from build123d import *

# Parameters (mm, degrees)
F0_R     = 7.5
F0_R_2   = 30
F1_DEPTH = 12
F2_R     = 3
F3_DEPTH = 20
F5_DEPTH = 20


with BuildPart() as f1:
    # F0 (on Right) → F1 (new body)
    with BuildSketch(Plane.YZ):
        with BuildLine():
            ThreePointArc((0, 32), (9.372583, 9.372583), (32, 0))
            Line((32, 0), (65, 0))
            ThreePointArc((65, 0), (68.535534, -1.464466), (70, -5))
            Line((70, -5), (70, -8.5))
            Line((70, -8.5), (202, -8.5))
            Line((202, -8.5), (202, 78.5))
            Line((202, 78.5), (70, 78.5))
            Line((70, 78.5), (70, 75))
            ThreePointArc((70, 75), (68.535534, 71.464466), (65, 70))
            Line((65, 70), (32, 70))
            ThreePointArc((32, 70), (9.372583, 60.627417), (0, 38))
            Line((0, 38), (0, 32))
        make_face()
        with Locations((32.5, 35)):
            Circle(F0_R, mode=Mode.SUBTRACT)
        with Locations((142, 35)):
            Circle(F0_R_2, mode=Mode.SUBTRACT)
    extrude(amount=F1_DEPTH)

    # F2 (on face) → F3 (cut)
    with BuildSketch(Plane.XY.offset(78.5)):
        with Locations((6, 80)):
            Circle(F2_R)
        with Locations((6, 110)):
            Circle(F2_R)
        with Locations((6, 140)):
            Circle(F2_R)
        with Locations((6, 170)):
            Circle(F2_R)
    extrude(amount=-F3_DEPTH, mode=Mode.SUBTRACT)

    # F4 (on face) → F5 (cut)
    with BuildSketch(Plane(origin=(0, 0, -8.5), x_dir=(1, 0, 0), z_dir=(0, 0, -1))):
        with BuildLine():
            ThreePointArc((6, -167), (3, -170), (6, -173))
            Line((6, -173), (6, -167))
        make_face()
        with BuildLine():
            ThreePointArc((6, -77), (3, -80), (6, -83))
            Line((6, -83), (6, -80))
            Line((6, -80), (6, -77))
        make_face()
        with BuildLine():
            Line((6, -80), (6, -83))
            ThreePointArc((6, -83), (8.12132, -82.12132), (9, -80))
            Line((9, -80), (6, -80))
        make_face()
        with BuildLine():
            ThreePointArc((6, -107), (3, -110), (6, -113))
            Line((6, -113), (6, -110))
            Line((6, -110), (6, -107))
        make_face()
        with BuildLine():
            Line((6, -110), (6, -113))
            ThreePointArc((6, -113), (8.12132, -112.12132), (9, -110))
            ThreePointArc((9, -110), (8.12132, -107.87868), (6, -107))
            Line((6, -107), (6, -110))
        make_face()
        with BuildLine():
            ThreePointArc((6, -137), (3, -140), (6, -143))
            Line((6, -143), (6, -137))
        make_face()
        with BuildLine():
            Line((6, -137), (6, -143))
            ThreePointArc((6, -143), (8.12132, -142.12132), (9, -140))
            ThreePointArc((9, -140), (8.12132, -137.87868), (6, -137))
        make_face()
        with BuildLine():
            Line((6, -167), (6, -173))
            ThreePointArc((6, -173), (8.12132, -172.12132), (9, -170))
            ThreePointArc((9, -170), (8.12132, -167.87868), (6, -167))
        make_face()
        with BuildLine():
            Line((6, -77), (6, -80))
            Line((6, -80), (9, -80))
            ThreePointArc((9, -80), (8.12132, -77.87868), (6, -77))
        make_face()
    extrude(amount=-F5_DEPTH, mode=Mode.SUBTRACT)


solid = f1.part
Geometry: final body of the model. Coordinates: model frame, mm. A direction names the side the tool comes from. Coordinates: 2 decimals unless noted, no trailing zeros. Loops run counter-clockwise (first coordinate to the right, second up) from the corner with the lowest first, then second, coordinate; pieces in that order, holes last. Notation, with made-up numbers: M -31,-30 L 20,-30 A29 ccw 20,-10 Z; hole C 50,62 d6. An arc over 180 degrees is marked long. One line per item, written item: value. Start each with the question number.
1) Cut plane C-C (z = 35). Return loops of the section in (x, y).
2) Cut plane A-A (z = 7.5). Return loops of the section in (x, y).
3) Draft query along Z for faces 1 (the cylindrical face through (5.92, 30.87, 27.68)), 2 (the cylindrical face through (3.6, 108.2, 68.6)), 3 (the flat face through (6, 49, 70)). Return one class per face: released by +Z, released by -Z, zero draft, split by the parting line, or undercut.
4) Reachability of faces 4 (the cylindrical face through (6, 173, 69)), 5 (the flat face through (6, 80, 11.5)), 6 (the flat face through (6, 48, 0)), 7 (the cylindrical face through (5.92, 9.62, 60.87)) from +Z, -Z, +X, -X, +Y, -Y: full face, straight path, thin tool, end or side. Return the list, or none.
5) Cut plane B-B (y = 153). Return loops of the section in (x, z).
6) Cut plane D-D (z = 22). Return loops of the section in (x, y).
7) Pin query (flat end, axial travel): P1, Ø3, axis at x = 7, z = 77, coming from the -Y side; P2, Ø6, axis at x = 8, y = 56.5, coming from the +Z side; P3, Ø5, axis at x = 6, y = 140, coming from the -Z side; P4, Ø5, axis at x = 6, y = 80, coming from the -Z side. Return the tip coordinate at first contact, or that it passes through.
8) Material intervals for L1, parallel to X at y = 140, z = 70.5; L2, parallel to Z at x = 7, y = 32.5; L3, parallel to Y at x = 9.25, z = 40, sorted ascending. Write a range as from..to.
Evaluation:
1. outline: M 0,0 L 12,0 L 12,25 L 0,25 Z; M 0,40 L 12,40 L 12,112 L 0,112 Z; M 0,172 L 12,172 L 12,202 L 0,202 Z
2. outline: M 0,11.41 L 12,11.41 L 12,130.01 L 0,130.01 Z; M 0,153.99 L 12,153.99 L 12,202 L 0,202 Z; hole M 6,77 A3 ccw 9,80 A3 ccw 6,83 A3 ccw Z; hole M 6,107 A3 ccw 9,110 A3 ccw 6,113 A3 ccw Z; hole M 6,167 A3 ccw 9,170 A3 ccw 6,173 A3 ccw Z
3. face 1: undercut
3. face 2: zero draft
3. face 3: released by +Z
4. face 4: +Z
4. face 5: -Z
4. face 6: -Z, +X, -X, -Y
4. face 7: +Z, +X, -X, -Y
5. outline: M 0,-8.5 L 12,-8.5 L 12,7.09 L 0,7.09 Z; M 0,62.91 L 12,62.91 L 12,78.5 L 0,78.5 Z
6. outline: M 0,1.6 L 12,1.6 L 12,114.96 L 0,114.96 Z; M 0,169.04 L 12,169.04 L 12,202 L 0,202 Z
7. P1: y = 70
7. P2: z = 70
7. P3: through
7. P4: z = 11.5
8. L1: 0..3, 9..12
8. L2: 0..27.5, 42.5..70
8. L3: 0.06..26.91, 38.09..112.42, 171.58..202
